Part model, mm, in its own coordinate system. Face numbers are marked on the shaded views. A direction names the side the tool comes from. Give positions to 0.01 mm unless a question says otherwise; leave off trailing zeros. Write each loop counter-clockwise with the first axis right and the second up, starting at its lowest first coordinate (ties: lowest second). Pieces come first, ordered by that corner, then holes.
```python
from build123d import *

# Parameters (mm, degrees)
DRIVER_R            = 27.06751
DRIVER_R_2          = 25.29025
BOSS_EXTRUDE1_DEPTH = 80
BOSS_EXTRUDE2_START = 50
DRIVER_3_R          = 29.1211
DRIVER_3_R_2        = 27.06751
BOSS_EXTRUDE2_DEPTH = 180
BOSS_EXTRUDE3_START = 200
DRIVER_4_R          = 27.06751
DRIVER_4_R_2        = 25.29025
BOSS_EXTRUDE3_DEPTH = 91.12


with BuildPart() as part:
    # driver → Boss-Extrude1 (new body)
    with BuildSketch(Plane(origin=(0, 0, 0), x_dir=(1, 0, 0), z_dir=(0, 1, 0))):
        Circle(DRIVER_R)
        Circle(DRIVER_R_2, mode=Mode.SUBTRACT)
    extrude(amount=BOSS_EXTRUDE1_DEPTH)

    # driver<3> → Boss-Extrude2 (add)
    with BuildSketch(Plane(origin=(0, 0, 0), x_dir=(1, 0, 0), z_dir=(0, 1, 0)).offset(BOSS_EXTRUDE2_START)):
        Circle(DRIVER_3_R)
        Circle(DRIVER_3_R_2, mode=Mode.SUBTRACT)
    extrude(amount=BOSS_EXTRUDE2_DEPTH)

    # driver<4> → Boss-Extrude3 (add)
    with BuildSketch(Plane(origin=(0, 0, 0), x_dir=(1, 0, 0), z_dir=(0, 1, 0)).offset(BOSS_EXTRUDE3_START)):
        Circle(DRIVER_4_R)
        Circle(DRIVER_4_R_2, mode=Mode.SUBTRACT)
    extrude(amount=BOSS_EXTRUDE3_DEPTH)


solid = part.part
```
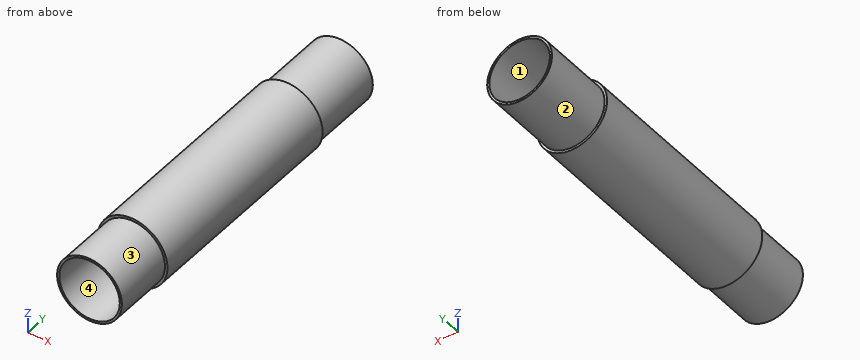
1) Wall check: L1, parallel to Z at x = 0, y = 53.5; L2, parallel to Z at x = 0, y = 108. Give the ranges that are in metal, low to high.
Answers follow:
L1: z = -29.12 to -25.29, 25.29 to 29.12
L2: z = -29.12 to -27.07, 27.07 to 29.12
2) Saw through at C-C, the plane y = 40.5. Write the cut outline in (x, z).
Answers follow:
outline: circle Ø54.14 at (0, 0); hole circle Ø50.58 at (0, 0)
3) Pin check, flat tips, straight feed: pin 1 Ø1.5 at (y, z) = (183, 8) entering from +X; pin 2 Ø6 at (y, z) = (200.5, 16.5) entering from +X; pin 3 Ø4 at (y, z) = (194.5, 11.5) entering from +X. Stop position of each tip, or through.
Answers follow:
pin 1: stops at x = 28.2
pin 2: stops at x = 25.8
pin 3: stops at x = 27.53
4) Two-plate mould, pull along Z, no slides. Class the marked faces 1 and 2: +Z half, -Z half, draft (parallel to the pull), parting line (faces both ways), or undercut.
Answers follow:
face 1: undercut
face 2: parting line
5) Saw through at A-A, the plane z = 0. Write the cut outline in (x, y).
Answers follow:
outline: (-29.12, 50) - (-27.07, 50) - (-27.07, 0) - (-25.29, 0) - (-25.29, 80) - (-27.07, 80) - (-27.07, 200) - (-25.29, 200) - (-25.29, 291.12) - (-27.07, 291.12) - (-27.07, 230) - (-29.12, 230) - close; (25.29, 0) - (27.07, 0) - (27.07, 50) - (29.12, 50) - (29.12, 230) - (27.07, 230) - (27.07, 291.12) - (25.29, 291.12) - (25.29, 200) - (27.07, 200) - (27.07, 80) - (25.29, 80) - close
6) 3-axis set-ups, long thin cutter, end or side, ignore diameter. For the marked faces 3 and 4: which of +Z, -Z, +X, -X, +Y, -Y reach the whole face in a straight line?
Answers follow:
face 3: -Y
face 4: +Y, -Y
7) Saw through at B-B, the plane x = 0. Write the cut outline in (y, z), then the cut area to 3 significant figures.
Answers follow:
outline: (0, -27.07) - (50, -27.07) - (50, -29.12) - (230, -29.12) - (230, -27.07) - (291.12, -27.07) - (291.12, -25.29) - (200, -25.29) - (200, -27.07) - (80, -27.07) - (80, -25.29) - (0, -25.29) - close; (0, 25.29) - (80, 25.29) - (80, 27.07) - (200, 27.07) - (200, 25.29) - (291.12, 25.29) - (291.12, 27.07) - (230, 27.07) - (230, 29.12) - (50, 29.12) - (50, 27.07) - (0, 27.07) - close
area: 1,350 mm2
